```python
from build123d import *

# Parameters (mm, degrees)
EXTRUDE_1_DEPTH     = 35
SKETCH_2_R          = 11
SKETCH_2_R_2        = 5
EXTRUDE_2_DEPTH     = 2
SKETCH_3_R          = 2.5
EXTRUDE_3_DEPTH     = 23
CUT_EXTRUDE_START   = -18
CUT_EXTRUDE_1_DEPTH = 18
SKETCH_5_R          = 1.5
CUT_EXTRUDE_2_DEPTH = 5


with BuildPart() as part:
    # 草图1 → 凸台-拉伸1 (new body)
    with BuildSketch(Plane.XY):
        Polygon((-17.183766184, 21), (17.183766184, 21), (21, 17.183766184), (21, -17.183766184), (17.183766184, -21), (-17.183766184, -21), (-21, -17.183766184), (-21, 17.183766184), align=None)
    extrude(amount=EXTRUDE_1_DEPTH)

    # 草图2 → 凸台-拉伸2 (add)
    with BuildSketch(Plane.XY.offset(35)):
        with Locations(Location((0, 0, 0), (0, 0, 180))):
            Circle(SKETCH_2_R)
        Circle(SKETCH_2_R_2, mode=Mode.SUBTRACT)
    extrude(amount=EXTRUDE_2_DEPTH)

    # 草图3 → 凸台-拉伸3 (add)
    with BuildSketch(Plane.XY.offset(35)):
        with Locations(Location((0, 0, 0), (0, 0, 180))):
            Circle(SKETCH_3_R)
    extrude(amount=EXTRUDE_3_DEPTH)

    # 草图4 → 切除-拉伸1 (cut)
    with BuildSketch(Plane.XY.offset(58).offset(CUT_EXTRUDE_START)):
        with BuildLine():
            Line((1.5, -2), (-1.5, -2))
            ThreePointArc((-1.5, -2), (0, -2.5), (1.5, -2))
        make_face()
    extrude(amount=CUT_EXTRUDE_1_DEPTH, mode=Mode.SUBTRACT)

    # 草图5 → 切除-拉伸2 (cut)
    with BuildSketch(Plane.XY.offset(35)):
        with Locations((-15.5, 15.5)):
            Circle(SKETCH_5_R)
        with Locations((15.5, 15.5)):
            Circle(SKETCH_5_R)
        with Locations((15.5, -15.5)):
            Circle(SKETCH_5_R)
        with Locations((-15.5, -15.5)):
            Circle(SKETCH_5_R)
    extrude(amount=-CUT_EXTRUDE_2_DEPTH, mode=Mode.SUBTRACT)


solid = part.part
```
The listing builds one solid part. Answer for the finished solid, in the listing's coordinates (mm). A direction names the side the tool comes from. Round coordinates to 2 decimals unless told otherwise and drop trailing zeros. Loops run counter-clockwise (first coordinate to the right, second up) from the corner with the lowest first, then second, coordinate; pieces in that order, holes last.
1) For a pull along Y with two mould halves and no side action, classify faces 3 (the face through (0, 21, 17)), 4 (the face through (15, -15, 30)), 5 (the face through (0, 0, 58)), 6 (the face through (-16, -15, 30)) as released by +Y, released by -Y, zero draft, split by the parting line, or undercut.
Outcome:
face 3: released by +Y
face 4: undercut
face 5: zero draft
face 6: undercut
2) A cutting plane is placed at D-D on y = 0. Determine the outline of the cut face in (x, z).
Outcome:
outline: (-21, 0) - (21, 0) - (21, 35) - (11, 35) - (11, 37) - (5, 37) - (5, 35) - (2.5, 35) - (2.5, 58) - (-2.5, 58) - (-2.5, 35) - (-5, 35) - (-5, 37) - (-11, 37) - (-11, 35) - (-21, 35) - close
3) A cutting plane is placed at C-C on z = 25.5. Determine the outline of the cut face in (x, y), plus the area to 3 significant figures.
Outcome:
outline: (-21, -17.18) - (-17.18, -21) - (17.18, -21) - (21, -17.18) - (21, 17.18) - (17.18, 21) - (-17.18, 21) - (-21, 17.18) - close
area: 1,730 mm2
4) Consider line 1 (Y direction, x = 15.5, z = 31.55); line 2 (Y direction, x = 0, z = 35.95); line 3 (X direction, y = 15, z = 33). Determine where each line is inside the solid, lowest interval first.
Outcome:
line 1: y = -21 to -17, -14 to 14, 17 to 21
line 2: y = -11 to -5, -2.5 to 2.5, 5 to 11
line 3: x = -21 to -16.91, -14.09 to 14.09, 16.91 to 21
5) A cutting plane is placed at B-B on x = 0. Determine the outline of the cut face in (y, z).
Outcome:
outline: (-21, 0) - (21, 0) - (21, 35) - (11, 35) - (11, 37) - (5, 37) - (5, 35) - (2.5, 35) - (2.5, 58) - (-2, 58) - (-2, 40) - (-2.5, 40) - (-2.5, 35) - (-5, 35) - (-5, 37) - (-11, 37) - (-11, 35) - (-21, 35) - close
6) For faces 1 (the face through (-2, -2, 35)), 2 (the face through (21, 0, 17)), determine the directions among +Z, -Z, +X, -X, +Y, -Y from which every point of the face is accessible in a straight line to the end or side of a thin tool.
Outcome:
face 1: +Z
face 2: +Z, -Z, +X, +Y, -Y
7) A cutting plane is placed at A-A on y = 15.5. Determine the outline of the cut face in (x, z).
Outcome:
outline: (-21, 0) - (21, 0) - (21, 35) - (17, 35) - (17, 30) - (14, 30) - (14, 35) - (-14, 35) - (-14, 30) - (-17, 30) - (-17, 35) - (-21, 35) - close
8) Given P1, Ø2.5, axis at x = 15.5, y = 15.5, coming from the -Z side; P2, Ø1.5, axis at x = 0.5, z = 52.5, coming from the -Y side; P3, Ø1.8, axis at x = -15.5, y = -15.5, coming from the +Z side; P4, Ø1, axis at y = -1.5, z = 49, coming from the -X side, each flat-ended and moving along its own axis, determine where each tip first touches the part or whether it passes through.
Outcome:
P1: stops at z = 0
P2: stops at y = -2
P3: stops at z = 30
P4: stops at x = -2.29
